Check sheet for the modelled part. Datum: model origin and axes. Units: mm. Face numbers are marked on the shaded views. A direction names the side the tool comes from. Give positions to 0.01 mm unless a question says otherwise; leave off trailing zeros. Write each loop counter-clockwise with the first axis right and the second up, starting at its lowest first coordinate (ties: lowest second). Pieces come first, ordered by that corner, then holes. Notation, with made-up numbers: M -37.5,48.5 L -10.5,48.5 A17 cw -10.5,52.5 Z; hole C -40,1 d3. An arc over 180 degrees is marked long. Use CSV: the item, a comma, the result in double quotes. Start each with the question number.
1. Cross-section at A-A, the plane y = 30. Enter the section's corners in (x, z), and give its area (3 significant figures).
2. Depth check by flat-ended pin: P1, Ø3.5, axis at x = 53, y = 4, coming from the -Z side; P2, Ø13.5, axis at x = -52.5, y = -8.5, coming from the -Z side; P3, Ø3, axis at x = -9, y = -11, coming from the -Z side; P4, Ø12, axis at x = 37.5, z = -10, coming from the -Y side. Enter the tip coordinate at first touch or a pass-through.
3. Mould release check, pull along X, two halves, no side actions. Record for the marked faces 1, 2 and 3: +X half, -X half, draft (parallel to the pull), parting line (faces both ways), or undercut.
4. Cross-section at C-C, the plane x = -40.5. Enter the section's corners in (y, z).
5. Access from +Z, -Z, +X, -X, +Y, -Y to the whole of each face (thin tool, end or side, straight path). Record for the marked faces 4, 5, 6 and 7.
6. Cross-section at B-B, the plane z = -10. Enter the section's corners in (x, y), and give its area (3 significant figures).
7. Cross-section at D-D, the plane z = 2. Enter the section's corners in (x, y).
8. Scan lines: line 1 (X direction, y = -16, z = -10); line 2 (Z direction, x = -37, y = -7); line 3 (Z direction, x = -2.5, y = 9). Record each from-to range of solid material in increasing order.
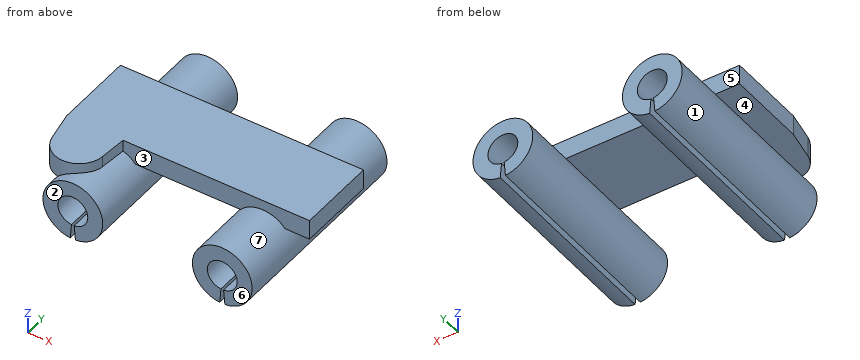
from build123d import *

# Parameters (mm, degrees)
F1_DEPTH = 10
F3_DEPTH = 50


with BuildPart() as f1:
    # F0 (on Top) → F1 (new body)
    with BuildSketch(Plane.XY):
        Polygon((-32.629684, -20), (61, -20), (61, 20), (-61, 20), (-61, -20), align=None)
        with BuildLine():
            Line((-33.740249, -33.694233), (-32.629684, -20))
            Line((-32.629684, -20), (-61, -20))
            Line((-61, -20), (-58.073841, -35.047843))
            ThreePointArc((-58.073841, -35.047843), (-45.316841, -44.981014), (-33.740249, -33.694233))
        make_face()
    extrude(amount=F1_DEPTH)

    # F2 (on Front) → F3 (join, symmetric)
    with BuildSketch(Plane.XZ):
        with BuildLine():
            ThreePointArc((36.846332, -17.47146), (37.5, -2.5), (38.153668, -17.47146))
            Line((38.153668, -17.47146), (38.807336, -24.94292))
            ThreePointArc((38.807336, -24.94292), (37.5, 5), (36.192664, -24.94292))
            Line((36.192664, -24.94292), (36.846332, -17.47146))
        make_face()
        with BuildLine():
            Line((-38.807336, -24.94292), (-38.153668, -17.47146))
            ThreePointArc((-38.153668, -17.47146), (-37.5, -2.5), (-36.846332, -17.47146))
            Line((-36.846332, -17.47146), (-36.192664, -24.94292))
            ThreePointArc((-36.192664, -24.94292), (-37.5, 5), (-38.807336, -24.94292))
        make_face()
    extrude(amount=F3_DEPTH, both=True)


solid = f1.part
Worked answers:
1,outline,"M -38.81,-24.94 L -38.15,-17.47 A7.5 cw long -36.85,-17.47 L -36.19,-24.94 A15 ccw long Z; M 36.19,-24.94 L 36.85,-17.47 A7.5 cw long 38.15,-17.47 L 38.81,-24.94 A15 ccw long Z"
1,area,"1,030 mm^2"
2,P1,"stops at z = -15.99"
2,P2,"stops at z = -22.53"
2,P3,"stops at z = 0"
2,P4,"passes through"
3,face 1,"undercut"
3,face 2,"draft"
3,face 3,"undercut"
4,outline,"M -50,-24.7 L 50,-24.7 L 50,-16.87 L -50,-16.87 Z; M -50,-3.13 L 50,-3.13 L 50,4.7 L 20,4.7 L 20,10 L -43.7,10 L -43.7,4.7 L -50,4.7 Z"
5,face 4,"-X, +Y, -Y"
5,face 5,"+Z, +Y"
5,face 6,"+Z, -Z, +X, -X, -Y"
5,face 7,"none"
6,outline,"M -52.5,-50 L -45,-50 L -45,50 L -52.5,50 Z; M -30,-50 L -22.5,-50 L -22.5,50 L -30,50 Z; M 22.5,-50 L 30,-50 L 30,50 L 22.5,50 Z; M 45,-50 L 52.5,-50 L 52.5,50 L 45,50 Z"
6,area,"3,000 mm^2"
7,outline,"M -61,-20 L -58.07,-35.05 A12.3 ccw -46.5,-44.99 L -46.5,-50 L -28.5,-50 L -28.5,-20 L 28.5,-20 L 28.5,-50 L 46.5,-50 L 46.5,-20 L 61,-20 L 61,20 L 46.5,20 L 46.5,50 L 28.5,50 L 28.5,20 L -28.5,20 L -28.5,50 L -46.5,50 L -46.5,20 L -61,20 Z"
8,line 1,"x = -52.5 to -45, -30 to -22.5, 22.5 to 30, 45 to 52.5"
8,line 2,"z = -2.52 to 10"
8,line 3,"z = 0 to 10"
